from build123d import *

# Parameters (mm, degrees)
F2_R     = 1.5
F3_DEPTH = 4.501


with BuildPart() as f1:
    # F0 (on Top) → F1 (revolve)
    with BuildSketch(Plane.XY):
        with BuildLine():
            Line((2.5, 11), (2.5, 0))
            Line((2.5, 0), (4.5, 0))
            Line((4.5, 0), (4.5, 5.625))
            ThreePointArc((4.5, 5.625), (3.5, 7.75), (4.5, 9.875))
            Line((4.5, 9.875), (4.5, 11))
            Line((4.5, 11), (2.5, 11))
        make_face()
    revolve(axis=Axis((0, 5.5, 0), (0, 1, 0)))

    # F2 (on Top) → F3 (cut, through all)
    with BuildSketch(Plane.XY):
        with Locations((0, 3)):
            Circle(F2_R)
    extrude(amount=F3_DEPTH, mode=Mode.SUBTRACT)


solid = f1.part
The listing builds one solid part. Answer for the finished solid, in the listing's coordinates (mm). A direction names the side the tool comes from. Give positions to 0.01 mm unless a question says otherwise; leave off trailing zeros. Write each loop counter-clockwise with the first axis right and the second up, starting at its lowest first coordinate (ties: lowest second). Pieces come first, ordered by that corner, then holes. Notation, with made-up numbers: (6.5, 73.25) - (42.5, 73.25) arc R19 cw to (42.5, 109.25) - close; hole circle Ø9 at (32.5, 12.25). An arc over 180 degrees is marked (long way). Use a Markdown table: item, result.
1. Find the intervals of material crossed by probe 1 along X at (y, z) = (5.25, 0); probe 2 along Z at (x, y) = (0, 3.5); probe 3 along Y at (x, z) = (0, 3.75), in increasing order. Write a range as from..to.
Values follow:
| item | result |
|---|---|
| probe 1 | x = -4.5..-2.5, 2.5..4.5 |
| probe 2 | z = -4.5..-2.5 |
| probe 3 | y = 0..1.5, 4.5..6.6, 8.9..11 |
2. Section D-D on z = 3.75 is taken. Count the separate pieces of the cut face and the enclosed holes in it, plus the area to 3 significant figures.
Values follow:
| item | result |
|---|---|
| separate pieces | 2 |
| enclosed holes | 1 |
| area | 32.2 mm² |
3. Section A-A on x = 0 is taken. Write down the section's boundary in (y, z) (3 decimals), plus the area to 3 significant figures.
Values follow:
| item | result |
|---|---|
| outline | (0, -4.5) - (5.625, -4.5) arc R2.758 cw to (9.875, -4.5) - (11, -4.5) - (11, -2.5) - (0, -2.5) - close; (0, 2.5) - (1.5, 2.5) - (1.5, 4.5) - (0, 4.5) - close; (4.5, 2.5) - (11, 2.5) - (11, 4.5) - (9.875, 4.5) arc R2.758 cw to (5.625, 4.5) - (4.5, 4.5) - close |
| area | 32.1 mm² |
4. For a pull along Z with two mould halves and no side action, classify faces 1 (the flat face through (-2, 0, 2)), 2 (the cylindrical face through (-0.59, 2.85, -4.46)), 3 (the cylindrical face through (-0.33, 5.42, -2.48)) as released by +Z, released by -Z, zero draft, split by the parting line, or undercut.
Values follow:
| item | result |
|---|---|
| face 1 | zero draft |
| face 2 | split by the parting line |
| face 3 | undercut |
5. Section C-C on y = 1.25 is taken. Write down the section's boundary in (x, z).
Values follow:
| item | result |
|---|---|
| outline | circle Ø9 at (0, 0); hole circle Ø5 at (0, 0) |
6. Each of these flat-tipped pins is pushed along its axis until it touches: P1, Ø4, axis at x = -2, y = 9, coming from the -Z side; P2, Ø4, axis at x = 3, z = 1.5, coming from the -Y side; P3, Ø1.5, axis at x = 3.5, y = 10, coming from the +Z side; P4, Ø3, axis at y = 8, z = -3, coming from the -X side. Where does it stop, or does it pass through?
Values follow:
| item | result |
|---|---|
| P1 | stops at z = -4.5 |
| P2 | stops at y = 0 |
| P3 | stops at z = 3.56 |
| P4 | stops at x = -3.31 |
7. A tool of negligible diameter and unlimited length cuts with its end or side. For faces 4 (the cylindrical face through (0.806, 4.265, 3.233)), 5 (the cylindrical face through (-0.59, 10.45, -4.46)), from which of +Z, -Z, +X, -X, +Y, -Y can it reach the whole face along a straight path? Write none if from no direction.
Values follow:
| item | result |
|---|---|
| face 4 | +Z |
| face 5 | +Y, -Y |
8. Section B-B on z = 0 is taken. Write down the section's boundary in (x, y) (3 decimals), plus the area to 3 significant figures.
Values follow:
| item | result |
|---|---|
| outline | (-4.5, 0) - (-2.5, 0) - (-2.5, 11) - (-4.5, 11) - (-4.5, 9.875) arc R2.758 cw to (-4.5, 5.625) - close; (2.5, 0) - (4.5, 0) - (4.5, 5.625) arc R2.758 cw to (4.5, 9.875) - (4.5, 11) - (2.5, 11) - close |
| area | 38.1 mm² |
